Model file for the job. Use its own axes, mm. Round coordinates to 2 decimals unless told otherwise and drop trailing zeros. Order: outer loops, then holes, each group sorted by start corner. A loop starts at its lowest first (then second) coordinate and runs counter-clockwise, first axis right, second up. Notation, with made-up numbers: (87.25, 40) - (130.25, 40) arc R22 ccw to (130.25, 57) - close; hole circle Ø1 at (73.5, 62). An arc over 180 degrees is marked (long way). Write item = value, one per line.
```python
from build123d import *

# Parameters (mm, degrees)
REVOLUTION001_ANGLE   = 180
CLONE_PLACEMENT_ANGLE = 180
PAD001_DEPTH          = 3.2


with BuildPart() as obj1:
    # Sketch001 → Revolution001 (revolve)
    with BuildSketch(Plane(origin=(3.195, 0.005, 0), x_dir=(0, 1, 0), z_dir=(1, 0, 0))):
        with BuildLine():
            Line((0, 4.24), (-1, 4.24))
            ThreePointArc((-1, 4.24), (-1.707107, 3.947107), (-2, 3.24))
            Line((-2, 3.24), (-2, 1.48))
            ThreePointArc((-2.2, 1.28), (-2.058579, 1.338579), (-2, 1.48))
            Line((-2.2, 1.28), (-2.2, 0.64))
            Line((-2.2, 0.64), (0, 0.64))
            Line((0, 4.24), (0, 0.64))
        make_face()
    revolve(axis=Axis((3.195, 0.005, 0), (0, 0, 1)), revolution_arc=REVOLUTION001_ANGLE)


with BuildPart() as clone:
    # Clone base: copy of obj1
    add(obj1.part)


with BuildPart() as clone_1:
    # Clone placement: moved
    add(clone.part.moved(Location((0, 0, 0))).rotate(Axis((0, 0, 0), (0, 0, 1)), CLONE_PLACEMENT_ANGLE))


with BuildPart() as pad001:
    # Sketch002 → Pad001 (new body, symmetric)
    with BuildSketch(Plane.YZ):
        with BuildLine():
            Line((0, 4.24), (-1, 4.24))
            ThreePointArc((-1, 4.24), (-1.707107, 3.947107), (-2, 3.24))
            Line((-2, 3.24), (-2, 1.48))
            ThreePointArc((-2.2, 1.28), (-2.058579, 1.338579), (-2, 1.48))
            Line((-2.2, 1.28), (-2.2, 0.64))
            Line((-2.2, 0.64), (0, 0.64))
            Line((0, 4.24), (0, 0.64))
        make_face()
    extrude(amount=PAD001_DEPTH, both=True)


with BuildPart() as obj2:
    # Part__Mirroring: instance of Pad001
    add(pad001.part.mirror(Plane(origin=(0, 0, 0), x_dir=(1, 0, 0), z_dir=(0, 1, 0))))

    # Fusion: union Pad001
    add(pad001.part)

    # Fusion001: union Clone, obj1
    add(clone_1.part)
    add(obj1.part)


solid = obj2.part
```
1) Wall check: line 1 along Y through (x, z) = (3.25, 1.5); line 2 along Y through (x, z) = (-1.25, 1.2); line 3 along X through (y, z) = (1, 1.45). Give the ranges that are in metal, low to high.
Conclusion:
line_1 = -1.99 to 2
line_2 = -2.2 to 2.2
line_3 = -4.93 to 4.93
2) Flat gauge pins, fed straight in: pin 1 Ø0.5 at (x, z) = (-1, 2) entering from -Y; pin 2 Ø1.3 at (y, z) = (2, 3) entering from -X; pin 3 Ø0.5 at (x, z) = (0, 2.5) entering from +Y. Where does each tip first touch, or does it go through?
Conclusion:
pin_1 = -2
pin_2 = -4.67
pin_3 = 2
3) Cut at B-B (x = 2). Write the cut outline in (y, z).
Conclusion:
outline = (-2.2, 0.64) - (2.2, 0.64) - (2.2, 1.28) arc R0.2 cw to (2, 1.48) - (2, 3.24) arc R1 ccw to (1, 4.24) - (-1, 4.24) arc R1 ccw to (-2, 3.24) - (-2, 1.48) arc R0.2 cw to (-2.2, 1.28) - close
4) Cut at A-A (z = 0.9). Write the cut outline in (x, y) (3 decimals).
Conclusion:
outline = (-3.2, 2.195) arc R2.2 ccw to (-3.195, -2.205) - (-3.195, -2.2) - (3.2, -2.2) - (3.2, -2.195) arc R2.2 ccw to (3.195, 2.205) - (3.195, 2.2) - (-3.2, 2.2) - close
5) Cut at C-C (z = 2). Write the cut outline in (x, y) (3 decimals).
Conclusion:
outline = (-3.2, 1.995) arc R2 ccw to (-3.195, -2.005) - (-3.195, -2) - (3.2, -2) - (3.2, -1.995) arc R2 ccw to (3.195, 2.005) - (3.195, 2) - (-3.2, 2) - close
